Input: part model. Units: mm. Frame: model coordinates. Face numbers are marked on the shaded views. A direction names the side the tool comes from. Coordinates: 2 decimals unless noted, no trailing zeros. Loops run counter-clockwise (first coordinate to the right, second up) from the corner with the lowest first, then second, coordinate; pieces in that order, holes last.
Item 1: Ray query, line 1 along Y through (x, z) = (341, -33.5); line 2 along Y through (x, z) = (277.5, -2.5); line 3 along X through (y, z) = (202, -29.5). Return the intervals inside material, ascending.
Item 2: Section C-C on z = -35. Give the number of separate pieces and of enclosed holes in the cut face, and give its area (3 significant figures).
Item 3: Section A-A on z = -8.5. Return loops of the section in (x, y), and give its area (3 significant figures).
Item 4: Reachability of the marked faces 1, 2 and 3 from +Z, -Z, +X, -X, +Y, -Y: full face, straight path, thin tool, end or side. Return the list, or none.
Item 5: Section B-B on y = -55.5. Return loops of the section in (x, z).
Item 6: Contact query for flat-ended pins moving along their axis: P1, Ø6, axis at x = 358.5, z = -38, coming from the +Y side; P2, Ø3, axis at x = 229.5, z = -25, coming from the +Y side; P3, Ø3, axis at y = 223.5, z = -29, coming from the -X side. Output: stop coordinate, or through.
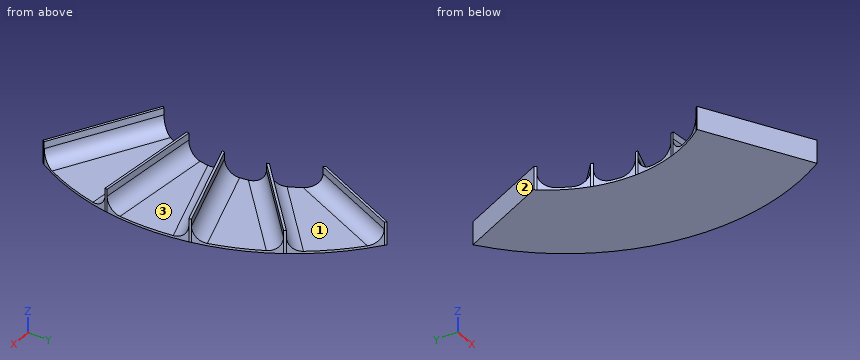
```python
from build123d import *

# Parameters (mm, degrees)
F1_DEPTH = 50
F2_DEPTH = 45
F3_R     = 30


with BuildPart() as f1:
    # F0 (on Top) → F1 (new body)
    with BuildSketch(Plane.XY):
        with BuildLine():
            ThreePointArc((194.916758, -97.186199), (194.096086, -99.609017), (193.25323, -102.024207))
            Line((193.25323, -102.024207), (419.168146, -128.763))
            ThreePointArc((419.168146, -128.763), (419.586918, -126.295419), (419.993217, -123.825754))
            Line((419.993217, -123.825754), (194.916758, -97.186199))
        make_face()
        with BuildLine():
            Line((419.168146, -128.763), (193.25323, -102.024207))
            ThreePointArc((193.25323, -102.024207), (176.040994, -140.915536), (153.116385, -176.738139))
            Line((153.116385, -176.738139), (356.739258, -297.881018))
            ThreePointArc((356.739258, -297.881018), (395.712182, -216.186004), (419.168146, -128.763))
        make_face()
        with BuildLine():
            Line((356.739258, -297.881018), (153.116385, -176.738139))
            ThreePointArc((153.116385, -176.738139), (151.592629, -178.742138), (150.050848, -180.732305))
            Line((150.050848, -180.732305), (354.182793, -302.17805))
            Line((354.182793, -302.17805), (356.739258, -297.881018))
        make_face()
        with BuildLine():
            ThreePointArc((209.125815, -17.369315), (204.936498, -57.796725), (194.916758, -97.186199))
            Line((194.916758, -97.186199), (419.993217, -123.825754))
            ThreePointArc((419.993217, -123.825754), (426.318532, -38.112086), (417.732158, 47.404677))
            Line((417.732158, 47.404677), (209.125815, -17.369315))
        make_face()
        with BuildLine():
            ThreePointArc((209.235921, -12.099633), (209.193315, -14.734734), (209.125815, -17.369315))
            Line((209.125815, -17.369315), (417.732158, 47.404677))
            ThreePointArc((417.732158, 47.404677), (417.258484, 49.874616), (416.772274, 52.342118))
            Line((416.772274, 52.342118), (209.235921, -12.099633))
        make_face()
        with BuildLine():
            ThreePointArc((198.100487, 69.182539), (206.672827, 28.953078), (209.235921, -12.099633))
            Line((209.235921, -12.099633), (416.772274, 52.342118))
            ThreePointArc((416.772274, 52.342118), (393.439703, 132.916412), (356.845379, 208.398073))
            Line((356.845379, 208.398073), (198.100487, 69.182539))
        make_face()
        with BuildLine():
            ThreePointArc((196.511281, 74.439195), (197.31882, 71.814778), (198.100487, 69.182539))
            Line((198.100487, 69.182539), (356.845379, 208.398073))
            ThreePointArc((356.845379, 208.398073), (355.541948, 210.578631), (354.227351, 212.752477))
            Line((354.227351, 212.752477), (196.511281, 74.439195))
        make_face()
        with BuildLine():
            ThreePointArc((152.708019, 159.463464), (178.280983, 118.842747), (196.511281, 74.439195))
            Line((196.511281, 74.439195), (354.227351, 212.752477))
            ThreePointArc((354.227351, 212.752477), (301.918092, 283.669214), (237.870183, 344.194478))
            Line((237.870183, 344.194478), (152.708019, 159.463464))
        make_face()
        with BuildLine():
            ThreePointArc((149.258975, 163.924782), (150.994771, 161.702839), (152.708019, 159.463464))
            Line((152.708019, 159.463464), (237.870183, 344.194478))
            Line((237.870183, 344.194478), (233.833063, 347.380159))
            Line((233.833063, 347.380159), (149.258975, 163.924782))
        make_face()
    extrude(amount=-F1_DEPTH)

    # F0 (on Top) → F2 (cut)
    with BuildSketch(Plane.XY):
        with BuildLine():
            Line((419.168146, -128.763), (193.25323, -102.024207))
            ThreePointArc((193.25323, -102.024207), (176.040994, -140.915536), (153.116385, -176.738139))
            Line((153.116385, -176.738139), (356.739258, -297.881018))
            ThreePointArc((356.739258, -297.881018), (395.712182, -216.186004), (419.168146, -128.763))
        make_face()
        with BuildLine():
            ThreePointArc((209.125815, -17.369315), (204.936498, -57.796725), (194.916758, -97.186199))
            Line((194.916758, -97.186199), (419.993217, -123.825754))
            ThreePointArc((419.993217, -123.825754), (426.318532, -38.112086), (417.732158, 47.404677))
            Line((417.732158, 47.404677), (209.125815, -17.369315))
        make_face()
        with BuildLine():
            ThreePointArc((198.100487, 69.182539), (206.672827, 28.953078), (209.235921, -12.099633))
            Line((209.235921, -12.099633), (416.772274, 52.342118))
            ThreePointArc((416.772274, 52.342118), (393.439703, 132.916412), (356.845379, 208.398073))
            Line((356.845379, 208.398073), (198.100487, 69.182539))
        make_face()
        with BuildLine():
            ThreePointArc((152.708019, 159.463464), (178.280983, 118.842747), (196.511281, 74.439195))
            Line((196.511281, 74.439195), (354.227351, 212.752477))
            ThreePointArc((354.227351, 212.752477), (301.918092, 283.669214), (237.870183, 344.194478))
            Line((237.870183, 344.194478), (152.708019, 159.463464))
        make_face()
    extrude(amount=-F2_DEPTH, mode=Mode.SUBTRACT)

    # F3
    f3_edges = [f1.edges().sort_by_distance(p)[0] for p in [
        (195.289101, 251.828971, -45),
        (275.369316, 143.595836, -45),
        (313.004098, 20.121242, -45),
        (307.454988, -110.505976, -45),
        (254.927822, -237.309578, -45),
        (277.472933, 138.790306, -45),
        (313.428987, 15.017681, -45),
        (306.210688, -115.393603, -45),
    ]]
    fillet(f3_edges, radius=F3_R)


solid = f1.part
```
Results found:
1. line 1: y = -294.34 to -281.09, -125.94 to -108.05, 16.89 to 35.5, 186.01 to 209.64
1. line 2: y = -256.56 to -250.74, -112 to -106.96, 3.86 to 9.1, 138.81 to 145.46
1. line 3: x = 166.81 to 176.43, 336.3 to 355.22
2. separate pieces: 5
2. enclosed holes: 0
2. area: 18,900 mm2
3. outline: (149.26, 163.92) arc R278.94 cw to (152.71, 159.46) - (237.87, 344.19) - (233.83, 347.38) - close; (150.05, -180.73) - (354.18, -302.18) - (356.74, -297.88) - (153.12, -176.74) arc R278.95 cw to start; (193.25, -102.02) - (419.17, -128.76) arc R495.36 ccw to (419.99, -123.83) - (194.92, -97.19) arc R278.94 cw to start; (196.51, 74.44) arc R278.95 cw to (198.1, 69.18) - (356.85, 208.4) arc R495.37 ccw to (354.23, 212.75) - close; (209.13, -17.37) - (417.73, 47.4) arc R495.27 ccw to (416.77, 52.34) - (209.24, -12.1) arc R278.95 cw to start
3. area: 5,480 mm2
4. face 1: +Z
4. face 2: +Z, -Z, -X, +Y
4. face 3: +Z, +X
5. outline: (205.34, -50) - (426.24, -50) - (426.24, -45) - (205.34, -45) - close
6. P1: stops at y = 210.65
6. P2: stops at y = 341.23
6. P3: stops at x = 176.03
